Autodesk Fusion 360 part; units mm, degrees
sketch "Sketch1" plane through (0, 0, 0) normal (0, 1, 0) x (1, 0, 0)
  circle A0 centre (0, 0) radius 17.5
  circle A1 centre (0, 0) radius 4
  dimension "d1" = 35
  dimension "d4" = 8
extrude "Extrude1" add sketch "Sketch1" along normal blind 5 makes body 1
sketch "Sketch2" plane through (0, 0, 0) normal (0, 1, 0) x (1, 0, 0)
  line L0 (17.5, 10) -> (117.5, 10)
  line L1 (117.5, 10) -> (117.5, -10)
  line L2 (117.5, -10) -> (17.5, -10)
  line L3 (17.5, -10) -> (17.5, 10)
  line L4 (17.5, 10) -> (117.5, -10) construction
  line L5 (117.5, 10) -> (17.5, -10) construction
  circle A0 centre (0, 0) radius 17.5
  point P0 (67.5, 0)
  dimension "d5" = 100
  dimension "d6" = 20
extrude "Extrude2" add sketch "Sketch2" along normal up to surface (5 mm away) separate body contours L0 L1 L2 L3 makes body 2
sketch "Sketch3" plane through (0, 5, 0) normal (0, 1, 0) x (-1, 0, 0)
  circle A0 centre (0, 0) radius 4
  circle A1 centre (0, 0) radius 17.5
  circle A2 centre (0, 0) radius 9.5
  circle A3 centre (0, 0) radius 8
  circle A4 centre (5.6569, -5.6569) radius 1.5
  circle A5 centre (-5.6569, 5.6569) radius 1.5
  circle A6 centre (6.7175, 6.7175) radius 1.5
  circle A7 centre (-6.7175, -6.7175) radius 1.5
  line L0 (0, 0) -> (-6.7175, -6.7175)
  line L1 (0, 0) -> (5.6569, -5.6569)
  line L2 (0, 0) -> (6.7175, 6.7175)
  line L3 (0, 0) -> (-5.6569, 5.6569)
  line L4 (0, 0) -> (-4, 0)
  dimension "d11" = 19
  dimension "d12" = 16
  dimension "d13" = 3
  dimension "d14" = 3
  dimension "d15" = 3
  dimension "d16" = 3
  dimension "d17" = 45
  dimension "d19" = 45
  dimension "d20" = 45
  dimension "d39" = 45
extrude "Extrude3" cut sketch "Sketch3" against normal blind 5 contours A2 A6 L2 | A2 A6 L2 | A3 A4 L1 | A3 A4 L1 | A3 A5 L3 | A3 A5 L3 | A3 A5 | A2 A6 | A2 A7 L0 | A2 A7 L0 | A3 A4 | A2 A7 bodies 1
sketch "Sketch4" plane through (0, 5, 0) normal (0, 1, 0) x (-1, 0, 0)
  line L0 (-17.5, -10) -> (-17.5, 10)
  line L1 (-17.5, 10) -> (-117.5, 10)
  line L2 (-117.5, 10) -> (-117.5, -10)
  line L3 (-117.5, -10) -> (-17.5, -10)
  arc A0 (-17.5, -10) -> (0, -17.5) centre (-1.8213, 2.4169) ccw
  arc A1 (0, 17.5) -> (-17.5, 10) centre (-1.8213, -2.4169) ccw
  line L4 (0, 17.5) -> (-15, 0)
  line L5 (-15, 0) -> (0, -17.5)
  dimension "d26" = 17.5
  dimension "d28" = 17.5
  dimension "d29" = 20
  dimension "d30" = 20
sketch "Sketch5" plane through (0, 5, 0) normal (0, 1, 0) x (-1, 0, 0)
  line L0 (-17.5, -10) -> (-17.5, 10)
  line L1 (-17.5, 10) -> (-117.5, 10)
  line L2 (-117.5, 10) -> (-117.5, -10)
  line L3 (-117.5, -10) -> (-17.5, -10)
  line L4 (-17.5, -10) -> (-12.5, -10)
  line L5 (-12.5, -10) -> (-12.5, 10)
  line L6 (-12.5, 10) -> (-17.5, 10)
  line L7 (-17.5, 10) -> (-17.5, -10)
  dimension "d33" = 5
extrude "Extrude5" add sketch "Sketch5" against normal blind 5 contours L0 L4 L5 L6 L7 bodies 1 2
fillet "Fillet1" radius 15 2 edges at (14.3614, 2.5, 10) (14.3614, 2.5, -10) on bodies 1
equation "d26 = ( 35 / 2 ) * 1 mm"
Geometry: final body of the model. Coordinates: model frame, mm. A direction names the side the tool comes from. Round coordinates to 2 decimals unless told otherwise and drop trailing zeros. Order: outer loops, then holes, each group sorted by start corner. A loop starts at its lowest first (then second) coordinate and runs counter-clockwise, first axis right, second up. Notation, with made-up numbers: (57, 19.5) - (105, 19.5) arc R18 cw to (105, 40.5) - close; hole circle Ø6 at (22, -19). An arc over 180 degrees is marked (long way). Use CSV: the item, a comma, the result in double quotes. Start each with the question number.
Q1. Section query A-A (z = 0). Return loops of the section in (x, y), and give its area (3 significant figures).
Q2. Material intervals for line 1 along Z through (x, y) = (-0.5, 4.15); line 2 along X through (y, z) = (2.4, 0.5); line 3 along Z through (x, y) = (51, 3.35), sorted ascending. Write a range as from..to.
Q3. Section query C-C (y = 2.75). Return loops of the section in (x, z), and give its area (3 significant figures).
Q4. Access query for faces 1 (the face through (70, 2, 10)), 2 (the face through (5.852, 2.535, 7.144)). Directions: +Z, -Z, +X, -X, +Y, -Y. A direction counts if a zero-diameter tool reaches every point of the face in a straight line with its end or side. Return the directions, or none.
Q5. Section query B-B (x = 0). Return loops of the section in (y, z), and give its area (3 significant figures).
Q6. Mould query, pull axis Z, two halves, no side actions, for faces 3 (the face through (68, 2, -10)), 4 (the face through (5.287, 2.535, -6.267)), 5 (the face through (49, 0, 0)), 6 (the face through (-0.867, 2.465, -3.905)). Classes: +Z half, -Z half, draft (parallel to the pull), parting line (faces both ways), or undercut.
Q7. First-contact query: pin 1 (1.5 mm diameter, centred on x = 91.5, y = 2.5, fed in from -Z); pin 2 (7 mm diameter, centred on x = 0, z = 0, fed in from +Y). Flat tips, straight axial feed; report the tip coordinate or a pass-through.
Q8. Section query D-D (x = 71.5). Return loops of the section in (y, z), and give its area (3 significant figures).
Result set:
1,outline,"(-17.5, 0) - (-4, 0) - (-4, 5) - (-17.5, 5) - close; (4, 0) - (117.5, 0) - (117.5, 5) - (4, 5) - close"
1,area,"635 mm2"
2,line 1,"z = -17.49..-3.97, 3.97..17.49"
2,line 2,"x = -17.49..-3.97, 3.97..117.5"
2,line 3,"z = -10..10"
3,outline,"(11.18, -13.46) arc R15 cw to (20.77, -10) - (117.5, -10) - (117.5, 10) - (20.77, 10) arc R15 cw to (11.18, 13.46) arc R17.5 ccw (long way) to start; hole circle Ø3 at (-6.72, 6.72); hole circle Ø3 at (-5.66, -5.66); hole circle Ø8 at (0, 0); hole circle Ø3 at (5.66, 5.66); hole circle Ø3 at (6.72, -6.72)"
3,area,"2,910 mm2"
4,face 1,"+Z, +X, +Y, -Y"
4,face 2,"+Y, -Y"
5,outline,"(0, -17.5) - (5, -17.5) - (5, -4) - (0, -4) - close; (0, 4) - (5, 4) - (5, 17.5) - (0, 17.5) - close"
5,area,"135 mm2"
6,face 3,"-Z half"
6,face 4,"undercut"
6,face 5,"draft"
6,face 6,"undercut"
7,pin 1,"stops at z = -10"
7,pin 2,"passes through"
8,outline,"(0, -10) - (5, -10) - (5, 10) - (0, 10) - close"
8,area,"100 mm2"
